Design review of the part built by this model. Coordinates are the model's own, in mm. A direction names the side the tool comes from. Coordinates: 2 decimals unless noted, no trailing zeros. Write each loop counter-clockwise with the first axis right and the second up, starting at its lowest first coordinate (ties: lowest second). Pieces come first, ordered by that corner, then holes. Notation, with made-up numbers: (74.5, 23.25) - (95.5, 23.25) arc R15 cw to (95.5, 36.25) - close; hole circle Ø1 at (41.5, 35). An arc over 180 degrees is marked (long way). Answer as a JSON object with one key per item and string values.
```python
from build123d import *

# Parameters (mm, degrees)
F0_R      = 10
F1_DEPTH  = 161
F3_W      = 160
F3_H      = 40
F4_DEPTH  = 5
F6_W      = 160
F6_H      = 40
F7_DEPTH  = 5
F8_SIZE   = 10
F10_D     = 8
F12_D     = 11
F12_DEPTH = 30
F12_TIP   = 3.3047334047


with BuildPart() as f1:
    # F0 (on Right) → F1 (new body)
    with BuildSketch(Plane.YZ):
        Circle(F0_R)
    extrude(amount=F1_DEPTH)

    # F3 (on offset) → F4 (join)
    with BuildSketch(Plane.YZ.offset(5)):
        with Locations((60, 0)):
            Rectangle(F3_W, F3_H)
    extrude(amount=F4_DEPTH)

    # F6 (on offset) → F7 (join)
    with BuildSketch(Plane.YZ.offset(50)):
        with Locations((60, -9.313e-07)):
            Rectangle(F6_W, F6_H)
    extrude(amount=F7_DEPTH)

    # F8
    f8_edges = [f1.edges().sort_by_distance(p)[0] for p in [
        (52.5, -20, 19.999999),
        (7.5, -20, 20),
        (7.5, -20, -20),
        (52.5, -20, -20.000001),
    ]]
    chamfer(f8_edges, length=F8_SIZE)

    # F10 (through all)
    with Locations(Plane(origin=(5, 0, 0), x_dir=(0, -1, 0), z_dir=(-1, 0, 0))):
        with Locations((-130, 0), (-80, 0), (-30, 0)):
            Hole(F10_D / 2)

    # F12
    with Locations(Plane.YZ.offset(161)):
        with Locations((0, 0)):
            Hole(F12_D / 2, depth=F12_DEPTH)
            with Locations((0, 0, -(F12_DEPTH + F12_TIP / 2))):  # 118° drill point
                Cone(0, F12_D / 2, F12_TIP, mode=Mode.SUBTRACT)


solid = f1.part
```
(1) To check wall thickness, follow line 1 (Z direction, x = 6.15, y = 80); line 2 (X direction, y = 66, z = 11); line 3 (Z direction, x = 150.25, y = 0). State the ranges of each line that lie inside material, in increasing order. Write a range as from..to.
Solved:
{"line 1": "z = -20..-4, 4..20", "line 2": "x = 5..10, 50..55", "line 3": "z = -10..-5.5, 5.5..10"}
(2) The part is to be moulded in two halves that separate along X. For faces 1 (the face through (161, 4, -4)), 2 (the face through (145.79, 1.19, -5.37)), 3 (the face through (0, 0, 0)), 4 (the face through (10, 59, 0)), say which applies: pulls with the +X half, pulls with the -X half, needs draft (parallel to the pull), parting line crosses it, or undercut.
Solved:
{"face 1": "pulls with the +X half", "face 2": "needs draft", "face 3": "pulls with the -X half", "face 4": "undercut"}
(3) Tool access review of faces 5 (the face through (2.46, -2.17, -9.76)), 6 (the face through (8, 76, 0)): name each direction out of +Z, -Z, +X, -X, +Y, -Y from which nothing blocks a thin tool from reaching the whole face with its end or side.
Solved:
{"face 5": "-X", "face 6": "+X, -X"}
(4) Take a section at D-D, the plane x = 32. Write out the cut boundary in (y, z).
Solved:
{"outline": "circle Ø20 at (0, 0)"}
(5) Take a section at B-B, the plane z = 13.5. Write out the cut boundary in (x, y), and give its area (4 significant figures).
Solved:
{"outline": "(5, -16.5) - (10, -16.5) - (10, 140) - (5, 140) - close; (50, -16.5) - (55, -16.5) - (55, 140) - (50, 140) - close", "area": "1,565 mm^2"}
(6) Take a section at C-C, the plane y = 66. Write out the cut boundary in (x, z).
Solved:
{"outline": "(5, -20) - (10, -20) - (10, 20) - (5, 20) - close; (50, -20) - (55, -20) - (55, 20) - (50, 20) - close"}
(7) For pin 1 (13 mm diameter, centred on y = 80, z = 0, fed in from +X); pin 2 (12 mm diameter, centred on y = 62, z = -4, fed in from -X), all flat-tipped, find the tip position at first contact; note any pin that passes through.
Solved:
{"pin 1": "stops at x = 55", "pin 2": "stops at x = 5"}
(8) Take a section at A-A, the plane y = 30. Write out the cut boundary in (x, z).
Solved:
{"outline": "(5, -20) - (10, -20) - (10, -4) - (5, -4) - close; (5, 4) - (10, 4) - (10, 20) - (5, 20) - close; (50, -20) - (55, -20) - (55, -4) - (50, -4) - close; (50, 4) - (55, 4) - (55, 20) - (50, 20) - close"}
